Here's the drawing with two shaded views (mm, measured from the low corner). I have some questions. Round coordinates to 2 decimals unless told otherwise and drop trailing zeros. Order: outer loops, then holes, each group sorted by start corner. A loop starts at its lowest first (then second) coordinate and runs counter-clockwise, first axis right, second up.
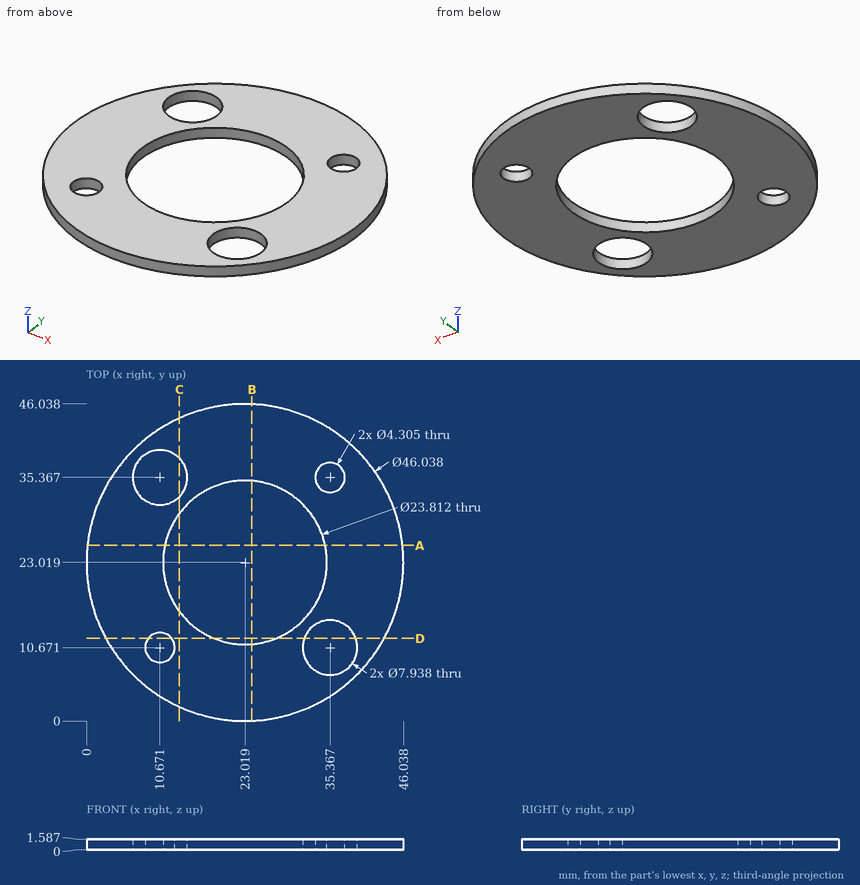
1. If we section it at C-C, the plane x = 13.5: Write out the boundary of the cut face in (y, z).
Evaluation:
outline: (2.06, 0) - (15.87, 0) - (15.87, 1.59) - (2.06, 1.59) - close; (30.17, 0) - (32.58, 0) - (32.58, 1.59) - (30.17, 1.59) - close; (38.15, 0) - (43.98, 0) - (43.98, 1.59) - (38.15, 1.59) - close
2. If we section it at D-D, the plane y = 12: Write out the boundary of the cut face in (x, z) (1 decimal).
Evaluation:
outline: (2.8, 0) - (9, 0) - (9, 1.6) - (2.8, 1.6) - close; (12.4, 0) - (18.5, 0) - (18.5, 1.6) - (12.4, 1.6) - close; (27.5, 0) - (31.6, 0) - (31.6, 1.6) - (27.5, 1.6) - close; (39.1, 0) - (43.2, 0) - (43.2, 1.6) - (39.1, 1.6) - close
3. I need wall thicknesses on probe 1 along Y at (x, z) = (23, 0.85) (1 decimal); probe 2 along X at (y, z) = (9, 0.2) (1 decimal). Which ranges of each line are inside material? Lowest first, please.
Evaluation:
probe 1: y = 0 to 11.1, 34.9 to 46
probe 2: x = 4.8 to 9.3, 12 to 31.8, 39 to 41.3
4. If we section it at A-A, the plane y = 25.5: Write out the boundary of the cut face in (x, z) (1 decimal).
Evaluation:
outline: (0.1, 0) - (11.4, 0) - (11.4, 1.6) - (0.1, 1.6) - close; (34.7, 0) - (45.9, 0) - (45.9, 1.6) - (34.7, 1.6) - close
5. If we section it at B-B, the plane x = 24: Write out the boundary of the cut face in (y, z) (1 decimal).
Evaluation:
outline: (0, 0) - (11.2, 0) - (11.2, 1.6) - (0, 1.6) - close; (34.9, 0) - (46, 0) - (46, 1.6) - (34.9, 1.6) - close
6. I'm going to push a flat-ended pin straight in: P1, Ø5, axis at x = 10.67, y = 35.37, coming from the +Z side. Where does the tip first touch, or does it pass through?
Evaluation:
P1: passes through
